Work out the finished part from the listing and answer in its coordinate system (mm). A direction names the side the tool comes from. Round coordinates to 2 decimals unless told otherwise and drop trailing zeros. Loops run counter-clockwise (first coordinate to the right, second up) from the corner with the lowest first, then second, coordinate; pieces in that order, holes last. Notation, with made-up numbers: (85.5, 47) - (104.5, 47) arc R33 cw to (104.5, 76) - close; hole circle Ø1 at (62.25, -17.5). An arc over 180 degrees is marked (long way). Return JSON: item names as keys, results as strings.
from build123d import *

# Parameters (mm, degrees)
F0_W     = 50
F0_H     = 50
F1_DEPTH = 10
F2_W     = 8
F2_H     = 30
F4_DEPTH = 40
F3_W     = 8
F3_H     = 30
F5_DEPTH = 40
F6_R     = 14.99999
F8_D     = 5
F9_DEPTH = 2


# Not quite as in the source:
# - a fillet or chamfer is up to 0.001 mm smaller than in the source, because OpenCascade refuses the exact size


with BuildPart() as f1:
    # F0 (on Top) → F1 (new body)
    with BuildSketch(Plane.XY):
        with Locations((-3.097159788, 1.3252983437)):
            Rectangle(F0_W, F0_H)
    extrude(amount=F1_DEPTH)

    # F2 (on face) → F4 (join)
    with BuildSketch(Plane.XY.offset(10)):
        with Locations((-14.097159788, 1.3252983437)):
            Rectangle(F2_W, F2_H)
    extrude(amount=F4_DEPTH)

    # F3 (on face) → F5 (join)
    with BuildSketch(Plane.XY.offset(10)):
        with Locations((7.902840212, 1.3252983437)):
            Rectangle(F3_W, F3_H)
    extrude(amount=F5_DEPTH)

    # F6 (radius 15 in the source; OpenCascade refuses exactly that, so slightly less here)
    f6_edges = [f1.edges().sort_by_distance(p)[0] for p in [
        (7.90284, -13.674702, 50),
        (7.90284, 16.325298, 50),
        (-14.09716, -13.674702, 50),
        (-14.09716, 16.325298, 50),
    ]]
    fillet(f6_edges, radius=F6_R)

    # F8 (through all)
    with Locations(Plane(origin=(-18.097159788, 0, 0), x_dir=(0, -1, 0), z_dir=(-1, 0, 0))):
        with Locations((-1.3252983437, 36.9870997965)):
            Hole(F8_D / 2)

    # F9 (add): a face of the model
    f9_faces = [f1.faces().sort_by_distance(p)[0] for p in [
        (-3.097159788, 1.3252983437, 10),
    ]]
    extrude(f9_faces, amount=F9_DEPTH)


solid = f1.part
1) Find the intervals of material crossed by L1, parallel to X at y = 10, z = 17; L2, parallel to Z at x = -3.5, y = -11.5; L3, parallel to Y at x = 11.5, z = 36, in increasing order.
Verdict:
{"L1": "x = -18.1 to -10.1, 3.9 to 11.9", "L2": "z = 0 to 12", "L3": "y = -13.64 to -0.97, 3.62 to 16.29"}
2) Section C-C (y = 20) is taken. Give the vertices of the cut face in (x, z).
Verdict:
{"outline": "(-28.1, 0) - (21.9, 0) - (21.9, 12) - (-28.1, 12) - close"}
3) Section D-D (z = 46) is taken. Give the vertices of the cut face in (x, y).
Verdict:
{"outline": "(-18.1, -8.87) - (-10.1, -8.87) - (-10.1, 11.52) - (-18.1, 11.52) - close; (3.9, -8.87) - (11.9, -8.87) - (11.9, 11.52) - (3.9, 11.52) - close"}
4) Determine the mould class of faces 4 (the flat face through (-28.097, 1, 6)), 5 (the flat face through (-10.097, 1, 31)), 6 (the flat face through (-3, 2, 0)) for opening direction X: pulls with the +X half, pulls with the -X half, needs draft (parallel to the pull), parting line crosses it, or undercut.
Verdict:
{"face 4": "pulls with the -X half", "face 5": "undercut", "face 6": "needs draft"}
5) A tool of negligible diameter and unlimited length cuts with its end or side. For faces 1 (the flat face through (-14, -13.675, 23)), 2 (the flat face through (-18.097, 1, 31)), 3 (the flat face through (3.903, 1, 31)), from which of +Z, -Z, +X, -X, +Y, -Y can it reach the whole face along a straight path? Write none if from no direction.
Verdict:
{"face 1": "+Z, +X, -X, -Y", "face 2": "+Z, -X, +Y, -Y", "face 3": "+Z, +Y, -Y"}
6) Section A-A (z = 28) is taken. Give the vertices of the cut face in (x, y), and give its area (3 significant figures).
Verdict:
{"outline": "(-18.1, -13.67) - (-10.1, -13.67) - (-10.1, 16.33) - (-18.1, 16.33) - close; (3.9, -13.67) - (11.9, -13.67) - (11.9, 16.33) - (3.9, 16.33) - close", "area": "480 mm2"}
7) Flat-ended cylindrical pins translate along their axes: pin 1 (9 mm diameter, centred on x = 9.5, z = 18.5, fed in from -Y); pin 2 (5 mm diameter, centred on y = 14.5, z = 12.5, fed in from -X); pin 3 (9 mm diameter, centred on y = 8, z = 29, fed in from -X); pin 4 (6 mm diameter, centred on y = -11.5, z = 34, fed in from +X). Find the tip coordinate at first contact, or state that the pin passes through.
Verdict:
{"pin 1": "stops at y = -13.67", "pin 2": "stops at x = -28.1", "pin 3": "stops at x = -18.1", "pin 4": "stops at x = 11.9"}
